```python
from build123d import *

# Parameters (mm, degrees)
BOSS_EXTRUDE1_DEPTH = 40
CUT_EXTRUDE1_REACH  = 99.98
SKETCH2_W           = 20
SKETCH2_H           = 10


with BuildPart() as part:
    # Sketch1 → Boss-Extrude1 (new body)
    with BuildSketch(Plane.XY):
        Polygon((0, 40), (0, 0), (80, 0), (80, 40), (50, 40), (50, 30), (65, 30), (65, 10), (15, 10), (15, 30), (30, 30), (30, 40), align=None)
    extrude(amount=BOSS_EXTRUDE1_DEPTH)

    # Sketch2 → Cut-Extrude1 (cut, up to next)
    with BuildSketch(Plane(origin=(80, 0, 0), x_dir=(0, 0, -1), z_dir=(1, 0, 0)), mode=Mode.PRIVATE) as cut_extrude1_sk1:
        with Locations((-30, 20)):
            Rectangle(SKETCH2_W, SKETCH2_H)
    cut_extrude1_tool1 = extrude(cut_extrude1_sk1.sketch, amount=-CUT_EXTRUDE1_REACH, mode=Mode.PRIVATE) & part.part
    add(cut_extrude1_tool1.solids().sort_by_distance((80, 20, 30))[0], mode=Mode.SUBTRACT)


solid = part.part
```
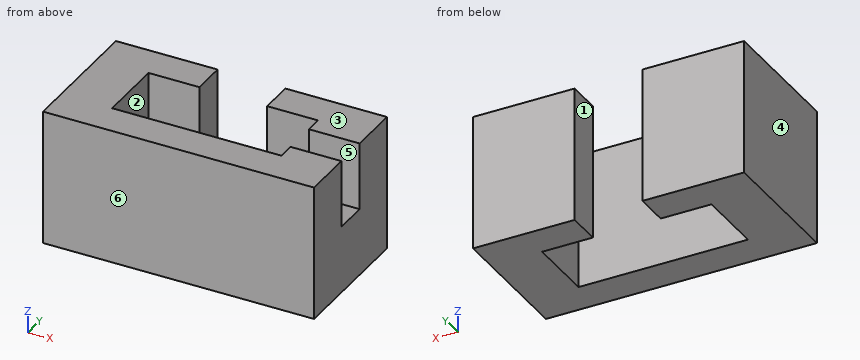
Here's how the part is built. I have some questions about the finished solid (model axes, mm). Face numbers are marked on the shaded views. A direction names the side the tool comes from. Give positions to 0.01 mm unless a question says otherwise; leave off trailing zeros. Loops run counter-clockwise (first coordinate to the right, second up) from the corner with the lowest first, then second, coordinate; pieces in that order, holes last. Notation, with made-up numbers: M -25,38 L -19,38 A14 ccw -19,54 Z; hole C 22,-6.5 d2. An arc over 180 degrees is marked long. Use one line per item in the form item = value. Start each with the question number.
Q1. I need wall thicknesses on line 1 along X through (y, z) = (36.5, 32.5); line 2 along Y through (x, z) = (62, 30.5); line 3 along Y through (x, z) = (73, 36). Which ranges of each line are inside material? Lowest first, please.
Q2. Which directions (+Z, -Z, +X, -X, +Y, -Y) give clear straight access to the entire face, cutting with the end or side of a thin tool? Please do the marked faces 1, 2 and 3.
Q3. If we section it at B-B (x = 56.5): Write out the boundary of the cut face in (y, z).
Q4. If we section it at A-A (y = 37.5): Write out the boundary of the cut face in (x, z).
Q5. Thinking about a two-plate mould opening in Y: for the marked faces 4, 5 and 6, which applies, +Y half, -Y half, draft (parallel to the pull), parting line (faces both ways), or undercut?
Q6. Will this pin go through, and if not, where does the flat tip stop? pin 1 Ø5 at (x, y) = (75.5, 20.5) entering from +Z.
Q7. If we section it at D-D (z = 4): Write out the boundary of the cut face in (x, y).
Q8. If we section it at C-C (z = 23.5): Write out the boundary of the cut face in (x, y), then the cut area to 3 significant figures.
Taken from the geometry:
q1.line_1 = 0 to 30, 50 to 80
q1.line_2 = 0 to 10, 30 to 40
q1.line_3 = 0 to 15, 25 to 40
q2.face_1 = +Z, -Z, +Y
q2.face_2 = +Z, -Z
q2.face_3 = +Z, +X, -X, +Y, -Y
q3.outline = M 0,0 L 10,0 L 10,40 L 0,40 Z; M 30,0 L 40,0 L 40,40 L 30,40 Z
q4.outline = M 0,0 L 30,0 L 30,40 L 0,40 Z; M 50,0 L 80,0 L 80,40 L 50,40 Z
q5.face_4 = draft
q5.face_5 = undercut
q5.face_6 = -Y half
q6.pin_1 = 20
q7.outline = M 0,0 L 80,0 L 80,40 L 50,40 L 50,30 L 65,30 L 65,10 L 15,10 L 15,30 L 30,30 L 30,40 L 0,40 Z
q8.outline = M 0,0 L 80,0 L 80,15 L 65,15 L 65,10 L 15,10 L 15,30 L 30,30 L 30,40 L 0,40 Z; M 50,30 L 65,30 L 65,25 L 80,25 L 80,40 L 50,40 Z
q8.area = 1,850 mm^2
